Work out the finished part from the listing and answer in its coordinate system (mm). A direction names the side the tool comes from. Coordinates: 2 decimals unless noted, no trailing zeros. Write each loop counter-clockwise with the first axis right and the second up, starting at its lowest first coordinate (ties: lowest second). Pieces come first, ordered by that corner, then holes. Notation, with made-up numbers: (59, 14.5) - (106, 14.5) arc R32 cw to (106, 51.5) - close; hole circle Ø10 at (-2.75, 1). An arc over 180 degrees is marked (long way). One line per item, written item: value.
```python
from build123d import *

# Parameters (mm, degrees)
F1_DEPTH = 4
F2_W     = 2.5
F2_H     = 2.5
F2_H_2   = 5.5
F2_W_2   = 2.75
F2_H_3   = 13.5
F2_H_4   = 11
F3_DEPTH = 2


with BuildPart() as f1:
    # F0 (on Top) → F1 (new body)
    with BuildSketch(Plane.XY):
        with BuildLine():
            Line((-64, 0), (0, 0))
            Line((0, 0), (0, 5))
            ThreePointArc((0, 5), (-4, 9), (0, 13))
            Line((0, 13), (0, 18))
            Line((0, 18), (-64, 18))
            Line((-64, 18), (-64, 0))
        make_face()
        with BuildLine():
            ThreePointArc((0, 13), (-4, 9), (0, 5))
            Line((0, 5), (0, 7))
            ThreePointArc((0, 7), (-2, 9), (0, 11))
            Line((0, 11), (0, 13))
        make_face()
        with BuildLine():
            Line((0, 7), (0, 5))
            ThreePointArc((0, 5), (2.8284271247, 6.1715728753), (4, 9))
            ThreePointArc((4, 9), (2.8284271247, 11.8284271247), (0, 13))
            Line((0, 13), (0, 11))
            ThreePointArc((0, 11), (1.4142135624, 10.4142135624), (2, 9))
            ThreePointArc((2, 9), (1.4142135624, 7.5857864376), (0, 7))
        make_face()
    extrude(amount=F1_DEPTH)

    # F2 (on face) → F3 (join)
    with BuildSketch(Plane.XY.offset(4)):
        with BuildLine():
            Line((-60.5, 17), (-63, 17))
            Line((-63, 17), (-63, 13))
            ThreePointArc((-63, 13), (-62.3166247904, 15.2360679775), (-60.5, 16.7080992435))
            Line((-60.5, 16.7080992435), (-60.5, 17))
        make_face()
        with BuildLine():
            ThreePointArc((-60.5, 9.2919007565), (-62.3166247904, 10.7639320225), (-63, 13))
            Line((-63, 13), (-63, 1))
            Line((-63, 1), (-60.5, 1))
            Line((-60.5, 1), (-60.5, 9.2919007565))
        make_face()
        with BuildLine():
            ThreePointArc((-60.5, 16.7080992435), (-62.3166247904, 15.2360679775), (-63, 13))
            ThreePointArc((-63, 13), (-62.3166247904, 10.7639320225), (-60.5, 9.2919007565))
            Line((-60.5, 9.2919007565), (-60.5, 13))
            Line((-60.5, 13), (-60.5, 16.7080992435))
        make_face()
        with BuildLine():
            ThreePointArc((-55, 13), (-56.7639320225, 16.3166247904), (-60.5, 16.7080992435))
            Line((-60.5, 16.7080992435), (-60.5, 13))
            Line((-60.5, 13), (-60.5, 9.2919007565))
            ThreePointArc((-60.5, 9.2919007565), (-56.7639320225, 9.6833752096), (-55, 13))
        make_face()
        with BuildLine():
            ThreePointArc((-57.5, 13), (-59, 11.5), (-60.5, 13))
            ThreePointArc((-60.5, 13), (-59, 14.5), (-57.5, 13))
        make_face(mode=Mode.SUBTRACT)
        with Locations((-52.75, 7.75)):
            Rectangle(F2_W, F2_H)
        with BuildLine():
            Line((-54, 13), (-54, 9))
            Line((-54, 9), (-51.5, 9))
            Line((-51.5, 9), (-51.5, 9.2919007565))
            ThreePointArc((-51.5, 9.2919007565), (-53.3166247904, 10.7639320225), (-54, 13))
        make_face()
        with Locations((-52.75, 3.75)):
            Rectangle(F2_W, F2_H_2)
        with BuildLine():
            ThreePointArc((-51.5, 16.7080992435), (-53.3166247904, 15.2360679775), (-54, 13))
            ThreePointArc((-54, 13), (-53.3166247904, 10.7639320225), (-51.5, 9.2919007565))
            Line((-51.5, 9.2919007565), (-51.5, 13))
            Line((-51.5, 13), (-51.5, 16.7080992435))
        make_face()
        Polygon((-50, 9), (-51.5, 9), (-51.5, 6.5), (-48.5, 6.5), (-48.5, 9), align=None)
        with BuildLine():
            ThreePointArc((-48.5, 16.7080992435), (-50, 17), (-51.5, 16.7080992435))
            Line((-51.5, 16.7080992435), (-51.5, 13))
            ThreePointArc((-51.5, 13), (-50, 14.5), (-48.5, 13))
            Line((-48.5, 13), (-48.5, 16.7080992435))
        make_face()
        with Locations((-47.25, 3.75)):
            Rectangle(F2_W, F2_H_2)
        with Locations((-47.25, 7.75)):
            Rectangle(F2_W, F2_H)
        with BuildLine():
            ThreePointArc((-46, 13), (-46.6833752096, 15.2360679775), (-48.5, 16.7080992435))
            Line((-48.5, 16.7080992435), (-48.5, 13))
            Line((-48.5, 13), (-48.5, 9.2919007565))
            ThreePointArc((-48.5, 9.2919007565), (-46.6833752096, 10.7639320225), (-46, 13))
        make_face()
        with BuildLine():
            Line((-48.5, 9.2919007565), (-48.5, 9))
            Line((-48.5, 9), (-46, 9))
            Line((-46, 9), (-46, 13))
            ThreePointArc((-46, 13), (-46.6833752096, 10.7639320225), (-48.5, 9.2919007565))
        make_face()
        with Locations((-43.625, 15.75)):
            Rectangle(F2_W_2, F2_H)
        with Locations((-41, 15.75)):
            Rectangle(F2_W, F2_H)
        with Locations((-38.375, 15.75)):
            Rectangle(F2_W_2, F2_H)
        with Locations((-41, 7.75)):
            Rectangle(F2_W, F2_H_3)
        with BuildLine():
            Line((-33.5, 17), (-36, 17))
            Line((-36, 17), (-36, 13))
            ThreePointArc((-36, 13), (-35.3166247904, 15.2360679775), (-33.5, 16.7080992435))
            Line((-33.5, 16.7080992435), (-33.5, 17))
        make_face()
        with BuildLine():
            ThreePointArc((-34.8284271247, 10.1715728753), (-35.69551813, 11.4692662705), (-36, 13))
            Line((-36, 13), (-36, 1))
            Line((-36, 1), (-33.5, 1))
            Line((-33.5, 1), (-33.5, 7.299987892))
            Line((-33.5, 7.299987892), (-34.8284271247, 10.1715728753))
        make_face()
        with BuildLine():
            ThreePointArc((-33.5, 16.7080992435), (-35.3166247904, 15.2360679775), (-36, 13))
            ThreePointArc((-36, 13), (-35.69551813, 11.4692662705), (-34.8284271247, 10.1715728753))
            ThreePointArc((-34.8284271247, 10.1715728753), (-34.2084555922, 9.6649252036), (-33.5, 9.2919007565))
            Line((-33.5, 9.2919007565), (-33.5, 13))
            Line((-33.5, 13), (-33.5, 16.7080992435))
        make_face()
        with BuildLine():
            ThreePointArc((-28, 13), (-29.7639320225, 16.3166247904), (-33.5, 16.7080992435))
            Line((-33.5, 16.7080992435), (-33.5, 13))
            ThreePointArc((-33.5, 13), (-32, 14.5), (-30.5, 13))
            ThreePointArc((-30.5, 13), (-31.4259748515, 11.6141807012), (-33.0606601718, 11.9393398282))
            Line((-33.0606601718, 11.9393398282), (-31.7058974503, 9.0108266909))
            ThreePointArc((-31.7058974503, 9.0108266909), (-29.0694360441, 10.2775388156), (-28, 13))
        make_face()
        with BuildLine():
            ThreePointArc((-33.5, 9.2919007565), (-34.2084555922, 9.6649252036), (-34.8284271247, 10.1715728753))
            Line((-34.8284271247, 10.1715728753), (-33.5, 7.299987892))
            Line((-33.5, 7.299987892), (-33.5, 9.2919007565))
        make_face()
        with BuildLine():
            ThreePointArc((-33.0606601718, 11.9393398282), (-33.3858192988, 12.4259748515), (-33.5, 13))
            Line((-33.5, 13), (-33.5, 9.2919007565))
            ThreePointArc((-33.5, 9.2919007565), (-32.6191105093, 9.048202665), (-31.7058974503, 9.0108266909))
            Line((-31.7058974503, 9.0108266909), (-33.0606601718, 11.9393398282))
        make_face()
        with BuildLine():
            ThreePointArc((-31.7058974503, 9.0108266909), (-32.6191105093, 9.048202665), (-33.5, 9.2919007565))
            Line((-33.5, 9.2919007565), (-33.5, 7.299987892))
            Line((-33.5, 7.299987892), (-30.5855555903, 1))
            Line((-30.5855555903, 1), (-28, 1))
            Line((-28, 1), (-31.7058974503, 9.0108266909))
        make_face()
        with Locations((-25.625, 15.75)):
            Rectangle(F2_W_2, F2_H)
        with Locations((-23, 15.75)):
            Rectangle(F2_W, F2_H)
        with Locations((-20.375, 15.75)):
            Rectangle(F2_W_2, F2_H)
        with Locations((-23, 9)):
            Rectangle(F2_W, F2_H_4)
        with Locations((-25.625, 2.25)):
            Rectangle(F2_W_2, F2_H)
        with Locations((-23, 2.25)):
            Rectangle(F2_W, F2_H)
        with Locations((-20.375, 2.25)):
            Rectangle(F2_W_2, F2_H)
        with BuildLine():
            ThreePointArc((-15.5, 9.2919007565), (-17.3166247904, 10.7639320225), (-18, 13))
            Line((-18, 13), (-18, 5))
            ThreePointArc((-18, 5), (-17.3166247904, 7.2360679775), (-15.5, 8.7080992435))
            Line((-15.5, 8.7080992435), (-15.5, 9.2919007565))
        make_face()
        with BuildLine():
            ThreePointArc((-15.5, 16.7080992435), (-17.3166247904, 15.2360679775), (-18, 13))
            ThreePointArc((-18, 13), (-17.3166247904, 10.7639320225), (-15.5, 9.2919007565))
            Line((-15.5, 9.2919007565), (-15.5, 13))
            Line((-15.5, 13), (-15.5, 16.7080992435))
        make_face()
        with BuildLine():
            ThreePointArc((-15.5, 8.7080992435), (-17.3166247904, 7.2360679775), (-18, 5))
            ThreePointArc((-18, 5), (-17.3166247904, 2.7639320225), (-15.5, 1.2919007565))
            Line((-15.5, 1.2919007565), (-15.5, 5))
            Line((-15.5, 5), (-15.5, 8.7080992435))
        make_face()
        with BuildLine():
            ThreePointArc((-10, 13), (-11.7639320225, 16.3166247904), (-15.5, 16.7080992435))
            Line((-15.5, 16.7080992435), (-15.5, 13))
            ThreePointArc((-15.5, 13), (-14, 14.5), (-12.5, 13))
            Line((-12.5, 13), (-10, 13))
        make_face()
        with BuildLine():
            Line((-15.5, 5), (-15.5, 1.2919007565))
            ThreePointArc((-15.5, 1.2919007565), (-11.7639320225, 1.6833752096), (-10, 5))
            Line((-10, 5), (-12.5, 5))
            ThreePointArc((-12.5, 5), (-14, 3.5), (-15.5, 5))
        make_face()
        Polygon((-6.5, 17), (-9, 17), (-9, 9), (-6.5, 12.6363636364), align=None)
        Polygon((-6.5, 5.3636363636), (-9, 9), (-9, 1), (-6.5, 1), align=None)
        Polygon((-6.5, 12.6363636364), (-9, 9), (-6.5, 5.3636363636), (-6.5, 9), align=None)
        Polygon((-3.5, 17), (-6.5, 12.6363636364), (-6.5, 9), (-1, 17), align=None)
        Polygon((-6.5, 9), (-6.5, 5.3636363636), (-3.5, 1), (-1, 1), align=None)
    extrude(amount=F3_DEPTH)


solid = f1.part
```
Item 1: Section A-A, the plane z = 1.6 is taken. Determine the outline of the cut face in (x, y).
Evaluation:
outline: (-64, 0) - (0, 0) - (0, 5) arc R4 ccw to (0, 13) - (0, 18) - (-64, 18) - close; hole circle Ø4 at (0, 9)
Item 2: Given pin 1 (3 mm diameter, centred on x = -24, z = 5, fed in from +Y); pin 2 (0.9 mm diameter, centred on x = -59, y = 13.5, fed in from +Z); pin 3 (0.6 mm diameter, centred on x = -41, z = 5.5, fed in from -Y); pin 4 (0.6 mm diameter, centred on y = 8, z = 5, fed in from -X), each flat-ended and moving along its own axis, determine where each tip first touches the part or whether it passes through.
Evaluation:
pin 1: stops at y = 18
pin 2: stops at z = 4
pin 3: stops at y = 1
pin 4: stops at x = -63
Item 3: Determine the mould class of faces 1 (the face through (-35, 1, 5)), 2 (the face through (-3.71, 4.94, 4.99)), 3 (the face through (-48.5, 11, 5)) for opening direction X: +X half, -X half, draft (parallel to the pull), parting line (faces both ways), or undercut.
Evaluation:
face 1: draft
face 2: +X half
face 3: undercut
Item 4: Section B-B, the plane x = -59 is taken. Determine the outline of the cut face in (y, z).
Evaluation:
outline: (0, 0) - (18, 0) - (18, 4) - (17, 4) - (17, 6) - (14.5, 6) - (14.5, 4) - (11.5, 4) - (11.5, 6) - (9, 6) - (9, 4) - (0, 4) - close
Item 5: Section C-C, the plane x = -34.5 is taken. Determine the outline of the cut face in (y, z).
Evaluation:
outline: (0, 0) - (18, 0) - (18, 4) - (17, 4) - (17, 6) - (1, 6) - (1, 4) - (0, 4) - close
Item 6: Which of the six approach directions +Z, -Z, +X, -X, +Y, -Y give full straight-line access (tool end or side, diameter ignored) to faces 4 (the face through (-53, 1, 5)), 5 (the face through (-11, 13, 5)), 6 (the face through (-38, 14.5, 5))?
Evaluation:
face 4: +Z, +X, -X, -Y
face 5: +Z
face 6: +Z, -Y
Item 7: Consider probe 1 along Y at (x, z) = (-59, 4.95); probe 2 along Z at (x, y) = (-29.5, 6); probe 3 along X at (y, z) = (10.5, 1.35). Determine where each line is inside the solid, lowest interval first.
Evaluation:
probe 1: y = 9 to 11.5, 14.5 to 17
probe 2: z = 0 to 4
probe 3: x = -64 to -1.32, 1.32 to 3.71
